from build123d import *
from build123d.topology import SkipClean

# Parameters (mm, degrees)
SKETCH_1_R      = 120
SKETCH_1_R_2    = 22.5
EXTRUDE_1_DEPTH = 10
EXTRUDE_START   = 40
SKETCH_2_R      = 32
SKETCH_2_R_2    = 22.5
EXTRUDE_2_DEPTH = 40
SKETCH_3_R      = 32
SKETCH_3_R_2    = 22.5
EXTRUDE_3_DEPTH = 5


with BuildPart() as part:
    # 草图1 → 凸台-拉伸1 (new body)
    with BuildSketch(Plane(origin=(0, 0, 0), x_dir=(1, 0, 0), z_dir=(0, 1, 0))):
        with Locations(Location((0, 0, 0), (0, 0, 270))):
            Circle(SKETCH_1_R)
        with Locations(Location((0, 0, 0), (0, 0, 270))):
            Circle(SKETCH_1_R_2, mode=Mode.SUBTRACT)
    extrude(amount=EXTRUDE_1_DEPTH)

    # 草图2 → 凸台-拉伸2 (add)
    with SkipClean():  # the faces are left unmerged after this step: merging them gives an invalid solid
        with BuildSketch(Plane.XZ.offset(EXTRUDE_START)):
            with Locations(Location((0, 0, 0), (0, 0, 90))):
                Circle(SKETCH_2_R)
            with Locations(Location((0, 0, 0), (0, 0, 270))):
                Circle(SKETCH_2_R_2, mode=Mode.SUBTRACT)
        extrude(amount=-EXTRUDE_2_DEPTH)

    # 草图3 → 凸台-拉伸3 (add)
    with BuildSketch(Plane(origin=(0, 10, 0), x_dir=(1, 0, 0), z_dir=(0, 1, 0))):
        with Locations(Location((0, 0, 0), (0, 0, 270))):
            Circle(SKETCH_3_R)
        with Locations(Location((0, 0, 0), (0, 0, 90))):
            Circle(SKETCH_3_R_2, mode=Mode.SUBTRACT)
    extrude(amount=EXTRUDE_3_DEPTH)


solid = part.part
Part model, mm, in its own coordinate system. A direction names the side the tool comes from. Coordinates: 2 decimals unless noted, no trailing zeros. Order: outer loops, then holes, each group sorted by start corner. A loop starts at its lowest first (then second) coordinate and runs counter-clockwise, first axis right, second up.
(1) Pin check, flat tips, straight feed: pin 1 Ø1 at (x, z) = (-62.5, 37) entering from +Y; pin 2 Ø1.5 at (x, z) = (61.5, -77.5) entering from -Y. Stop position of each tip, or through.
Check sheet entries:
pin 1: stops at y = 10
pin 2: stops at y = 0
(2) Slice it at A-A, the plane z = 0. Write the cut outline in (x, y), and give its area (4 significant figures).
Check sheet entries:
outline: (-120, 0) - (-32, 0) - (-32, -40) - (-22.5, -40) - (-22.5, 15) - (-32, 15) - (-32, 10) - (-120, 10) - close; (22.5, -40) - (32, -40) - (32, 0) - (120, 0) - (120, 10) - (32, 10) - (32, 15) - (22.5, 15) - close
area: 2,805 mm2
(3) Tool access for faces 1 (the face through (7, -40, -22)), 2 (the face through (31.24, -20.28, -6.94)), 3 (the face through (-31.24, 12.46, -6.94)): list every direction of +Z, -Z, +X, -X, +Y, -Y with a clear straight run to the whole face (end or side of a thin tool).
Check sheet entries:
face 1: +Z, -Z, +X, -X, -Y
face 2: -Y
face 3: +Y
(4) Slice it at D-D, the plane x = -77. Write the cut outline in (y, z), and give its area (3 significant figures).
Check sheet entries:
outline: (0, -92.04) - (10, -92.04) - (10, 92.04) - (0, 92.04) - close
area: 1,840 mm2
(5) Slice it at B-B, the plane x = 0. Write the cut outline in (y, z).
Check sheet entries:
outline: (-40, -32) - (0, -32) - (0, -120) - (10, -120) - (10, -32) - (15, -32) - (15, -22.5) - (-40, -22.5) - close; (-40, 22.5) - (15, 22.5) - (15, 32) - (10, 32) - (10, 120) - (0, 120) - (0, 32) - (-40, 32) - close
(6) Probe L1, parallel to X at y = 14, z = 0; L2, parallel to Z at x = 1, y = 1.5; L3, parallel to X at y = 2, z = 0. List the from-to ranges inside material, lowest first.
Check sheet entries:
L1: x = -32 to -22.5, 22.5 to 32
L2: z = -120 to -22.48, 22.48 to 120
L3: x = -120 to -22.5, 22.5 to 120
(7) Slice it at C-C, the plane y = -28. Write the cut outline in (x, z).
Check sheet entries:
outline: circle Ø64 at (0, 0); hole circle Ø45 at (0, 0)
